```python
from build123d import *

# Parameters (mm, degrees)
ESQUISSE1_W             = 600
ESQUISSE1_H             = 150
BOSS_EXTRU_1_DEPTH      = 18
ESQUISSE3_R             = 11
ENL_V_MAT_EXTRU_1_DEPTH = 20
ESQUISSE4_W             = 7
ESQUISSE4_H             = 14
ENL_V_MAT_EXTRU_2_DEPTH = 12


with BuildPart() as part:
    # Esquisse1 → Boss.-Extru.1 (new body)
    with BuildSketch(Plane(origin=(0, 0, 0), x_dir=(1, 0, 0), z_dir=(0, 1, 0))):
        Rectangle(ESQUISSE1_W, ESQUISSE1_H)
    extrude(amount=BOSS_EXTRU_1_DEPTH)

    # Esquisse3 → Enlèv. mat.-Extru.1 (cut)
    with BuildSketch(Plane(origin=(0, 18, 0), x_dir=(1, 0, 0), z_dir=(0, 1, 0))):
        with Locations(Location((269, -54, 0), (0, 0, 270))):
            Circle(ESQUISSE3_R)
        with Locations(Location((-269, -54, 0), (0, 0, 270))):
            Circle(ESQUISSE3_R)
    extrude(amount=-ENL_V_MAT_EXTRU_1_DEPTH, mode=Mode.SUBTRACT)

    # Esquisse4 → Enlèv. mat.-Extru.2 (cut)
    with BuildSketch(Plane(origin=(0, 18, 0), x_dir=(1, 0, 0), z_dir=(0, 1, 0))):
        with Locations((289, -58)):
            Rectangle(ESQUISSE4_W, ESQUISSE4_H)
    extrude(amount=-ENL_V_MAT_EXTRU_2_DEPTH, mode=Mode.SUBTRACT)


solid = part.part
```
Model file for the job. Use its own axes, mm. A direction names the side the tool comes from. Coordinates: 2 decimals unless noted, no trailing zeros. Loops run counter-clockwise (first coordinate to the right, second up) from the corner with the lowest first, then second, coordinate; pieces in that order, holes last. Notation, with made-up numbers: (-21, 65.5) - (12, 65.5) arc R19 ccw to (12, 71.5) - close; hole circle Ø3 at (-20, 16.5). An arc over 180 degrees is marked (long way). Write item = value, one per line. Start each with the question number.
Item 1: Drop flat-ended pins along their axis: pin 1 Ø1.5 at (x, z) = (-69.5, 29.5) entering from -Y; pin 2 Ø3.5 at (x, z) = (289, 61) entering from +Y; pin 3 Ø13 at (x, z) = (-269, 54) entering from -Y. Give the stop position or say it passes through.
Item 2: Saw through at A-A, the plane x = 269. List the corners of the cut face in (y, z).
Item 3: Pull direction X, two halves, no side cores. Call faces 3 (the face through (285.5, 12, 58)), 4 (the face through (-300, 9, 1)), 5 (the face through (-4, 0, -1)): +X half, -X half, draft (parallel to the pull), parting line (faces both ways), or undercut.
Item 4: Wall check: probe 1 along X at (y, z) = (13.5, 54); probe 2 along X at (y, z) = (15.75, 61). Give the ranges that are in metal, low to high. Write a range as [from, to].
Item 5: 3-axis set-ups, long thin cutter, end or side, ignore diameter. For faces 1 (the face through (292.5, 12, 58)), 2 (the face through (-4, 9, 75)): which of +Z, -Z, +X, -X, +Y, -Y reach the whole face in a straight line?
Answers:
q1.pin_1 = 0
q1.pin_2 = 6
q1.pin_3 = through
q2.outline = (0, -75) - (18, -75) - (18, 43) - (0, 43) - close; (0, 65) - (18, 65) - (18, 75) - (0, 75) - close
q3.face_3 = undercut
q3.face_4 = -X half
q3.face_5 = draft
q4.probe_1 = [-300, -280], [-258, 258], [280, 285.5], [292.5, 300]
q4.probe_2 = [-300, -277.49], [-260.51, 260.51], [277.49, 285.5], [292.5, 300]
q5.face_1 = +Y
q5.face_2 = +Z, +X, -X, +Y, -Y
